Autodesk Inventor part; units mm, degrees
ref_plane "YZ Plane" through (0, 0, 0) normal (1, 0, 0) x (0, 1, 0)
ref_plane "XZ Plane" through (0, 0, 0) normal (0, 1, 0) x (-1, 0, 0)
ref_plane "XY Plane" through (0, 0, 0) normal (0, 0, 1) x (1, 0, 0)
sketch "Náčrt1" plane through (0, 0, 0) normal (0, 0, 1) x (1, 0, 0)
  line L0 (70.5158, 9.6388) -> (-69.4838, 10)
  line L1 (70.5158, 9.6388) -> (137.3455, -37.1558)
  line L2 (70.5158, 9.6388) -> (152.0998, 9.6388) construction
  line L3 (137.3455, -37.1558) -> (125.874, -53.5389)
  line L4 (-69.4838, 10) -> (-136.3135, -36.7947)
  line L5 (-69.4838, 10) -> (12.1002, 10) construction
  line L6 (-136.3135, -36.7947) -> (-124.8419, -53.1777)
  line L7 (0.6215, 10) -> (0.5893, -2.5)
  line L8 (-124.8419, -53.1777) -> (0.5893, -2.5)
  line L9 (125.874, -53.5389) -> (0.5893, -2.5)
  point P0 (0, 0)
  dimension "d2" = 140
  dimension "d3" = 81.584
  dimension "d4" = 35
  dimension "d5" = 20
  dimension "d6" = 81.584
  dimension "d7" = 145
  dimension "d8" = 20
  dimension "d9" = 12.5
  dimension "d22" = 135.282
  dimension "d23" = 135.282
extrude "Vysunutí1" add sketch "Náčrt1" along normal blind 5
sketch "Náčrt2" plane through (0, 0, 5) normal (0, 0, 1) x (1, 0, 0)
  line L0 (-136.3135, -36.7947) -> (-124.8419, -53.1777)
  line L1 (-124.8419, -53.1777) -> (-101.6623, -43.8125)
  line L2 (-124.8419, -53.1777) -> (0.5893, -2.5)
  line L3 (-101.6623, -43.8125) -> (-111.5137, -19.4297)
  line L4 (-69.4838, 10) -> (-136.3135, -36.7947)
  line L5 (-136.3135, -36.7947) -> (-124.8419, -53.1777)
  line L6 (0.5893, -2.5) -> (125.874, -53.5389)
  line L7 (125.874, -53.5389) -> (102.7215, -44.1069)
  line L8 (102.7215, -44.1069) -> (112.6093, -19.8353)
  line L9 (137.3455, -37.1558) -> (70.5158, 9.6388)
  line L10 (137.3455, -37.1558) -> (112.6093, -19.8353)
  line L11 (125.874, -53.5389) -> (137.3455, -37.1558)
  line L12 (125.874, -53.5389) -> (137.3455, -37.1558)
  point P0 (0, 0)
  dimension "d12" = 25
  dimension "d13" = 25
extrude "Vysunutí2" cut sketch "Náčrt2" against normal blind 5
sketch "Náčrt5" plane through (0, 0, 5) normal (0, 0, 1) x (1, 0, 0)
  line L0 (70.5158, 9.6388) -> (-69.4838, 10)
  line L1 (-69.4838, 10) -> (-69.4838, 5)
  line L2 (-69.4838, 10) -> (-64.4838, 10) construction
  line L3 (112.6093, -19.8353) -> (70.5158, 9.6388)
  line L4 (70.5158, 9.6388) -> (70.5158, 4.6388)
  line L5 (70.5158, 9.6388) -> (75.5158, 9.6388) construction
  circle A0 centre (-69.4838, 5) radius 2
  circle A1 centre (70.5158, 4.6388) radius 2
  point P0 (0, 0)
  dimension "d24" = 5
  dimension "d25" = 90
  dimension "d26" = 5
  dimension "d27" = 90
  dimension "d28" = 4
  dimension "d29" = 4
extrude "Vysunutí4" cut sketch "Náčrt5" against normal blind 10
properties part number "zaver"
The listing builds one solid part. Answer for the finished solid, in the listing's coordinates (mm). A direction names the side the tool comes from. Coordinates: 2 decimals unless noted, no trailing zeros. Write each loop counter-clockwise with the first axis right and the second up, starting at its lowest first coordinate (ties: lowest second). Pieces come first, ordered by that corner, then holes.
Q1. Which of the six approach directions +Z, -Z, +X, -X, +Y, -Y give full straight-line access (tool end or side, diameter ignored) to faces 1 (the flat face through (52.37, -23.595, 2.465)), 2 (the flat face through (-1, 1, 5))?
Returned:
face 1: +Z, -Z, -Y
face 2: +Z, +X, -X, +Y, -Y
Q2. Given P1, Ø2.5, axis at x = 70.52, y = 4.64, coming from the +Z side; P2, Ø1.5, axis at y = -9, z = 1.5, coming from the +X side; P3, Ø3, axis at y = -19.5, z = 4, coming from the +X side; P4, Ø2, axis at y = -6.5, z = 0.5, coming from the +X side, each flat-ended and moving along its own axis, determine where each tip first touches the part or whether it passes through.
Returned:
P1: passes through
P2: stops at x = 98.21
P3: stops at x = 112.61
P4: stops at x = 94.99
Q3. Section C-C, the plane y = -35 is taken. Write down the section's boundary in (x, z).
Returned:
outline: (-105.22, 0) - (-79.85, 0) - (-79.85, 5) - (-105.22, 5) - close; (80.37, 0) - (106.43, 0) - (106.43, 5) - (80.37, 5) - close
Q4. The mould has two halves that part along Y. Classify faces 3 (the cylindrical face through (72.423, 5.24, 2.535)), 4 (the flat face through (-51.252, -23.445, 2.465)), 5 (the flat face through (91.268, -4.892, 2.465)): released by +Y, released by -Y, zero draft, split by the parting line, or undercut.
Returned:
face 3: undercut
face 4: released by -Y
face 5: released by +Y
Q5. Section A-A, the plane y = -9 is taken. Write down the section's boundary in (x, z), then the cut area to 3 significant figures.
Returned:
outline: (-96.62, 0) - (-15.5, 0) - (-15.5, 5) - (-96.62, 5) - close; (16.54, 0) - (97.13, 0) - (97.13, 5) - (16.54, 5) - close
area: 809 mm2
Q6. Section B-B, the plane z = 1.75 is taken. Write down the section's boundary in (x, y), then the cut area to 3 significant figures.
Returned:
outline: (-111.51, -19.43) - (-101.66, -43.81) - (0.59, -2.5) - (102.72, -44.11) - (112.61, -19.84) - (70.52, 9.64) - (-69.48, 10) - close; hole circle Ø4 at (-69.48, 5); hole circle Ø4 at (70.52, 4.64)
area: 6,310 mm2
Q7. Find the intervals of material crossed by line 1 along X through (y, z) = (4, 0.2); line 2 along X through (y, z) = (3.5, 2.9); line 3 along X through (y, z) = (-27, 2.65), in increasing order.
Returned:
line 1: x = -78.05 to -71.22, -67.75 to 68.62, 72.41 to 78.57
line 2: x = -78.77 to -70.81, -68.16 to 68.87, 72.16 to 79.28
line 3: x = -108.46 to -60.05, 60.73 to 109.69
Q8. Section D-D, the plane x = 51.5 is taken. Write down the section's boundary in (y, z).
Returned:
outline: (-23.24, 0) - (9.69, 0) - (9.69, 5) - (-23.24, 5) - close
